Build history of the part. All positions in model axes, mm. Coordinates: 2 decimals unless noted, no trailing zeros. Loops run counter-clockwise (first coordinate to the right, second up) from the corner with the lowest first, then second, coordinate; pieces in that order, holes last.
Item 1: Cut at C-C (x = -60). List the corners of the cut face in (y, z), and give its area (3 significant figures).
Item 2: Cut at A-A (z = -24). List the corners of the cut face in (x, y), and give its area (3 significant figures).
Item 3: Mould opens along X. For faces 1 (the face through (1, 2, 30)), 2 (the face through (75, 0, 0)), 3 (the face through (-58, 0, -24)), 4 (the face through (0, -2, -18)) say: released by +X, released by -X, zero draft, split by the parting line, or undercut.
Item 4: Drill centre lines: line 1 along X through (y, z) = (4, 24); line 2 along X through (y, z) = (0, 14); line 3 along X through (y, z) = (0, -22.5). Where is each one in solid material? Low to high.
Item 5: Cut at B-B (y = 0). List the corners of the cut face in (x, z) (3 decimals).
Item 6: Cut at D-D (z = 0). List the corners of the cut face in (x, y) (3 decimals), and give its area (3 significant figures).
from build123d import *

# Parameters (mm, degrees)
SKETCH1_R           = 5.975
SKETCH1_R_2         = 2
BOSS_EXTRUDE1_DEPTH = 7.5
SKETCH2_R           = 2
CUT_EXTRUDE1_DEPTH  = 97.33924434


with BuildPart() as part:
    # Sketch1 → Boss-Extrude1 (new, symmetric)
    with BuildSketch(Plane(origin=(0, 0, 0), x_dir=(1, 0, 0), z_dir=(0, 1, 0))):
        with BuildLine():
            Line((-73, 30), (73, 30))
            ThreePointArc((73, 30), (74.414213562, 29.414213562), (75, 28))
            Line((75, 28), (75, -28))
            ThreePointArc((75, -28), (74.414213562, -29.414213562), (73, -30))
            Line((73, -30), (-73, -30))
            ThreePointArc((-73, -30), (-74.414213562, -29.414213562), (-75, -28))
            Line((-75, -28), (-75, 28))
            ThreePointArc((-75, 28), (-74.414213562, 29.414213562), (-73, 30))
        make_face()
        with Locations(Location((0, 0, 0), (0, 0, 270))):
            Circle(SKETCH1_R, mode=Mode.SUBTRACT)
        with Locations(Location((-60, 24, 0), (0, 0, 270))):
            Circle(SKETCH1_R_2, mode=Mode.SUBTRACT)
        with Locations(Location((-60, -24, 0), (0, 0, 270))):
            Circle(SKETCH1_R_2, mode=Mode.SUBTRACT)
        with Locations(Location((60, -24, 0), (0, 0, 270))):
            Circle(SKETCH1_R_2, mode=Mode.SUBTRACT)
        with Locations(Location((60, 24, 0), (0, 0, 270))):
            Circle(SKETCH1_R_2, mode=Mode.SUBTRACT)
    extrude(amount=BOSS_EXTRUDE1_DEPTH, both=True)

    # Sketch2 → Cut-Extrude1 (cut, through all)
    with BuildSketch(Plane.XY.offset(30)):
        Circle(SKETCH2_R)
    extrude(amount=-CUT_EXTRUDE1_DEPTH, mode=Mode.SUBTRACT)


solid = part.part
Filled sheet:
1. outline: (-7.5, -30) - (7.5, -30) - (7.5, -26) - (-7.5, -26) - close; (-7.5, -22) - (7.5, -22) - (7.5, 22) - (-7.5, 22) - close; (-7.5, 26) - (7.5, 26) - (7.5, 30) - (-7.5, 30) - close
1. area: 780 mm2
2. outline: (-75, -7.5) - (-62, -7.5) - (-62, 7.5) - (-75, 7.5) - close; (-58, -7.5) - (58, -7.5) - (58, 7.5) - (-58, 7.5) - close; (62, -7.5) - (75, -7.5) - (75, 7.5) - (62, 7.5) - close; hole circle Ø4 at (0, 0)
2. area: 2,120 mm2
3. face 1: zero draft
3. face 2: released by +X
3. face 3: undercut
3. face 4: undercut
4. line 1: x = -75 to -62, -58 to 58, 62 to 75
4. line 2: x = -75 to -2, 2 to 75
4. line 3: x = -75 to -61.32, -58.68 to -2, 2 to 58.68, 61.32 to 75
5. outline: (-75, -28) arc R2 ccw to (-73, -30) - (-2, -30) - (-2, -5.63) arc R5.975 cw to (-2, 5.63) - (-2, 30) - (-73, 30) arc R2 ccw to (-75, 28) - close; (2, -30) - (73, -30) arc R2 ccw to (75, -28) - (75, 28) arc R2 ccw to (73, 30) - (2, 30) - (2, 5.63) arc R5.975 cw to (2, -5.63) - close; hole circle Ø4 at (-60, -24); hole circle Ø4 at (-60, 24); hole circle Ø4 at (60, -24); hole circle Ø4 at (60, 24)
6. outline: (-75, -7.5) - (-5.975, -7.5) - (-5.975, 7.5) - (-75, 7.5) - close; (5.975, -7.5) - (75, -7.5) - (75, 7.5) - (5.975, 7.5) - close
6. area: 2,070 mm2
